Design review of the part built by this model. Coordinates are the model's own, in mm. Face numbers are marked on the shaded views. A direction names the side the tool comes from. Give positions to 0.01 mm unless a question says otherwise; leave off trailing zeros. Loops run counter-clockwise (first coordinate to the right, second up) from the corner with the lowest first, then second, coordinate; pieces in that order, holes last. Notation, with made-up numbers: (11.25, 24.5) -> (25.25, 24.5) arc R31 cw to (25.25, 63.5) -> close; hole circle Ø5 at (-37.5, 65). An arc over 180 degrees is marked (long way). Answer as CSV lines item,"result".
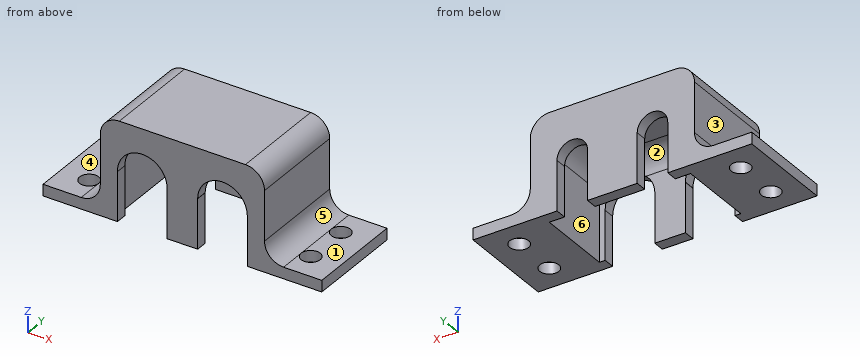
from build123d import *

# Parameters (mm, degrees)
F1_W          = 43
F1_H          = 26
F2_DEPTH      = 13
F2_DEPTH_BACK = 13
F3_T          = -3
F5_W          = 15
F5_H          = 26
F5_R          = 2.5
F5_W_2        = 43
F5_W_3        = 37
F5_H_2        = 20
F6_DEPTH      = 3
F7_R          = 4.99999
F9_DEPTH      = 5
F10_DEPTH     = 25


# Not quite as in the source:
# - a fillet or chamfer is up to 0.001 mm smaller than in the source, because OpenCascade refuses the exact size


with BuildPart() as f2:
    # F1 (on Top) → F2 (new body, two sides)
    with BuildSketch(Plane.XY) as f2_sk:
        with Locations((0, 13)):
            Rectangle(F1_W, F1_H)
    extrude(amount=F2_DEPTH)
    extrude(f2_sk.sketch, amount=-F2_DEPTH_BACK)

    # F3
    f3_openings = [f2.faces().sort_by_distance(p)[0] for p in [
        (0, 13, -13),
    ]]
    offset(amount=F3_T, openings=f3_openings)

    # F5 (on face) → F6 (join)
    with BuildSketch(Plane(origin=(0, 0, -13), x_dir=(1, 0, 0), z_dir=(0, 0, -1))):
        with Locations((-29, -13)):
            Rectangle(F5_W, F5_H)
        with Locations((-29, -19)):
            Circle(F5_R, mode=Mode.SUBTRACT)
        with Locations((-29, -7)):
            Circle(F5_R, mode=Mode.SUBTRACT)
        with Locations((0, -13)):
            Rectangle(F5_W_2, F5_H)
        with Locations((0, -13)):
            Rectangle(F5_W_3, F5_H_2, mode=Mode.SUBTRACT)
        with Locations((29, -13)):
            Rectangle(F5_W, F5_H)
        with Locations((29, -19)):
            Circle(F5_R, mode=Mode.SUBTRACT)
        with Locations((29, -7)):
            Circle(F5_R, mode=Mode.SUBTRACT)
    extrude(amount=-F6_DEPTH)

    # F7 (radius 5 in the source; OpenCascade refuses exactly that, so slightly less here)
    f7_edges = [f2.edges().sort_by_distance(p)[0] for p in [
        (-21.5, 13, 13),
        (21.5, 13, 13),
        (-21.5, 13, -10),
        (21.5, 13, -10),
        (0, 23, 10),
        (0, 3, 10),
        (-18.5, 13, 10),
        (18.5, 13, 10),
    ]]
    fillet(f7_edges, radius=F7_R)

    # F8 (on face) → F9 (cut)
    with BuildSketch(Plane.XZ):
        with BuildLine():
            Line((-4.0000936475, -11), (-4.0000936475, -0.0348913798))
            ThreePointArc((-4.0000936475, -0.0348913798), (-4, 0), (-4.0000936475, 0.0348913798))
            ThreePointArc((-4.0000936475, 0.0348913798), (-10.5909716955, 6.499363365), (-16.9983365331, -0.1470452389))
            Line((-16.9983365331, -0.1470452389), (-16.9983365331, -10.9773843356))
            Line((-16.9983365331, -10.9773843356), (-16.9983365331, -13))
            Line((-16.9983365331, -13), (-4.0000936475, -13))
            Line((-4.0000936475, -13), (-4.0000936475, -11))
        make_face()
        with BuildLine():
            ThreePointArc((4.0000936475, 0.0348913798), (4, 0), (4.0000936475, -0.0348913798))
            Line((4.0000936475, -0.0348913798), (4.0000936475, -11))
            Line((4.0000936475, -11), (4.0000936475, -13))
            Line((4.0000936475, -13), (16.9983365331, -13))
            Line((16.9983365331, -13), (16.9983365331, -10.9773843356))
            Line((16.9983365331, -10.9773843356), (16.9983365331, -0.1470452389))
            ThreePointArc((16.9983365331, -0.1470452389), (10.5909716955, 6.499363365), (4.0000936475, 0.0348913798))
        make_face()
    extrude(amount=-F9_DEPTH, mode=Mode.SUBTRACT)

    # F4 (on face) → F10 (cut)
    with BuildSketch(Plane(origin=(0, 26, 0), x_dir=(-1, 0, 0), z_dir=(0, 1, 0))):
        with BuildLine():
            Line((-6.5, -13), (-6.5, 0))
            ThreePointArc((-6.5, 0), (-10.5, 4), (-14.5, 0))
            Line((-14.5, 0), (-14.5, -13))
            Line((-14.5, -13), (-6.5, -13))
        make_face()
        with BuildLine():
            ThreePointArc((14.5, 0), (10.5, 4), (6.5, 0))
            Line((6.5, 0), (6.5, -13))
            Line((6.5, -13), (14.5, -13))
            Line((14.5, -13), (14.5, 0))
        make_face()
    extrude(amount=-F10_DEPTH, mode=Mode.SUBTRACT)


solid = f2.part
Q1. To check wall thickness, follow probe 1 along X at (y, z) = (19, -11.7); probe 2 along Y at (x, z) = (29, -12.05); probe 3 along X at (y, z) = (6.75, -2.5). State the ranges of each line that lie inside material, in increasing order. Write a range as from..to.
Filled sheet:
probe 1,"x = -36.5..-31.5, -26.5..-18.5, 18.5..26.5, 31.5..36.5"
probe 2,"y = 0..4.5, 9.5..16.5, 21.5..26"
probe 3,"x = -21.5..-18.5, 18.5..21.5"
Q2. We need section B-B, the plane x = 30.5. State the section outline as (y, z) points.
Filled sheet:
outline,"(0, -13) -> (5, -13) -> (5, -10) -> (0, -10) -> close; (9, -13) -> (17, -13) -> (17, -10) -> (9, -10) -> close; (21, -13) -> (26, -13) -> (26, -10) -> (21, -10) -> close"
Q3. For the marked faces 1, 2 and 3, list the 3-axis set-ups (+Z, -Z, +X, -X, +Y, -Y) from which the entire face can be reached by the end or side of a thin tool; tool diameter is ignored.
Filled sheet:
face 1,"+Z, +X, +Y, -Y"
face 2,"-Z"
face 3,"+Z, -X, +Y, -Y"
Q4. Clearance check with flat-ended pins moving along their axes: pin 1 Ø0.9 at (y, z) = (25, -7) entering from +X; pin 2 Ø1.5 at (y, z) = (1.5, -6.5) entering from -X; pin 3 Ø2.5 at (y, z) = (1.5, -5.5) entering from +X; pin 4 Ø4 at (x, y) = (29, 7) entering from +Z. State where each tip first meets the part, or that it passes through.
Filled sheet:
pin 1,"stops at x = 22.14"
pin 2,"stops at x = -22.03"
pin 3,"stops at x = 21.82"
pin 4,"passes through"
Q5. We need section C-C, the plane y = 13.25. State the section outline as (x, z) points, and give its area (3 significant figures).
Filled sheet:
outline,"(-36.5, -13) -> (-18.5, -13) -> (-18.5, 5) arc R5 cw to (-13.5, 10) -> (13.5, 10) arc R5 cw to (18.5, 5) -> (18.5, -13) -> (36.5, -13) -> (36.5, -10) -> (26.5, -10) arc R5 cw to (21.5, -5) -> (21.5, 8) arc R5 ccw to (16.5, 13) -> (-16.5, 13) arc R5 ccw to (-21.5, 8) -> (-21.5, -5) arc R5 cw to (-26.5, -10) -> (-36.5, -10) -> close"
area,"368 mm^2"
Q6. The part is to be moulded in two halves that separate along X. For the marked faces 4, 5 and 6, say which applies: pulls with the +X half, pulls with the -X half, needs draft (parallel to the pull), parting line crosses it, or undercut.
Filled sheet:
face 4,"needs draft"
face 5,"pulls with the +X half"
face 6,"undercut"
Q7. We need section D-D, the plane x = 10.5. State the section outline as (y, z) points, and give its area (3 significant figures).
Filled sheet:
outline,"(0, 6.5) -> (3.23, 6.5) arc R5 cw to (8, 10) -> (18, 10) arc R5 cw to (23, 5) -> (23, 4) -> (26, 4) -> (26, 13) -> (0, 13) -> close"
area,"117 mm^2"
Q8. We need section A-A, the plane z = -2. State the section outline as (x, y) points, and give its area (3 significant figures).
Filled sheet:
outline,"(-21.5, 0) -> (-17, 0) -> (-17, 3) -> (-18.5, 3) -> (-18.5, 23) -> (-14.5, 23) -> (-14.5, 26) -> (-21.5, 26) -> close; (-6.5, 23) -> (6.5, 23) -> (6.5, 26) -> (-6.5, 26) -> close; (-4, 0) -> (4, 0) -> (4, 3) -> (-4, 3) -> close; (14.5, 23) -> (18.5, 23) -> (18.5, 3) -> (17, 3) -> (17, 0) -> (21.5, 0) -> (21.5, 26) -> (14.5, 26) -> close"
area,"252 mm^2"
